Design review of the part built by this model. Coordinates are the model's own, in mm. A direction names the side the tool comes from. Round coordinates to 2 decimals unless told otherwise and drop trailing zeros. Order: outer loops, then holes, each group sorted by start corner. A loop starts at its lowest first (then second) coordinate and runs counter-clockwise, first axis right, second up. Notation, with made-up numbers: (27.5, -22.5) - (86.5, -22.5) arc R13 cw to (86.5, -3.5) - close; hole circle Ø10 at (-0.5, -25.75). An arc over 180 degrees is marked (long way). Write item = value, one per line.
from build123d import *

# Parameters (mm, degrees)
CROQUIS2_W              = 110
CROQUIS2_H              = 75
CROQUIS2_R              = 2
CROQUIS2_R_2            = 1.997516107
SALIENTE_EXTRUIR1_DEPTH = 15
CROQUIS3_R              = 4
CORTAR_EXTRUIR1_DEPTH   = 6
REDONDEO2_R             = 2
CROQUIS4_R              = 3.5
CROQUIS4_R_2            = 3
CORTAR_EXTRUIR8_DEPTH   = 15
CROQUIS5_R              = 3.701474701
SALIENTE_EXTRUIR2_DEPTH = 15
CROQUIS7_R              = 4
CROQUIS7_R_2            = 5
CORTAR_EXTRUIR9_DEPTH   = 15


with BuildPart() as part:
    # Croquis2 → Saliente-Extruir1 (new body)
    with BuildSketch(Plane.XY):
        with Locations((-693.862272549, 896.557366956)):
            Rectangle(CROQUIS2_W, CROQUIS2_H)
        with Locations((-741.862272549, 866.057366956)):
            Circle(CROQUIS2_R, mode=Mode.SUBTRACT)
        with Locations((-645.862272549, 866.057366956)):
            Circle(CROQUIS2_R, mode=Mode.SUBTRACT)
        with BuildLine():
            Line((-728.862272549, 925.057366956), (-706.362272549, 925.057366956))
            Line((-706.362272549, 925.057366956), (-681.362272549, 925.057366956))
            Line((-681.362272549, 925.057366956), (-658.862272549, 925.057366956))
            ThreePointArc((-658.862272549, 925.057366956), (-655.326738643, 923.592900862), (-653.862272549, 920.057366956))
            Line((-653.862272549, 920.057366956), (-653.862272549, 873.057366956))
            ThreePointArc((-653.862272549, 873.057366956), (-655.326738643, 869.52183305), (-658.862272549, 868.057366956))
            Line((-658.862272549, 868.057366956), (-681.362272549, 868.057366956))
            Line((-681.362272549, 868.057366956), (-706.362272549, 868.057366956))
            Line((-706.362272549, 868.057366956), (-728.862272549, 868.057366956))
            ThreePointArc((-728.862272549, 868.057366956), (-732.397806455, 869.52183305), (-733.862272549, 873.057366956))
            Line((-733.862272549, 873.057366956), (-733.862272549, 920.057366956))
            ThreePointArc((-733.862272549, 920.057366956), (-732.397806455, 923.592900862), (-728.862272549, 925.057366956))
        make_face(mode=Mode.SUBTRACT)
        with Locations((-741.862272549, 927.057366956)):
            Circle(CROQUIS2_R, mode=Mode.SUBTRACT)
        with Locations((-645.862272549, 927.057366956)):
            Circle(CROQUIS2_R_2, mode=Mode.SUBTRACT)
    extrude(amount=SALIENTE_EXTRUIR1_DEPTH)

    # Croquis3 → Cortar-Extruir1 (cut)
    with BuildSketch(Plane.XY.offset(15)):
        with Locations((-645.862272549, 927.057366956)):
            Circle(CROQUIS3_R)
        with Locations((-645.862272549, 866.057366956)):
            Circle(CROQUIS3_R)
        with Locations((-741.862272549, 866.057366956)):
            Circle(CROQUIS3_R)
        with Locations((-741.862272549, 927.057366956)):
            Circle(CROQUIS3_R)
    extrude(amount=-CORTAR_EXTRUIR1_DEPTH, mode=Mode.SUBTRACT)

    # Redondeo2
    redondeo2_edges = [part.edges().sort_by_distance(p)[0] for p in [
        (-693.862272549, 859.057366956, 15),
        (-693.862272549, 934.057366956, 15),
    ]]
    fillet(redondeo2_edges, radius=REDONDEO2_R)

    # Croquis4 → Cortar-Extruir8 (cut)
    with BuildSketch(Plane.XY.offset(15)):
        with Locations((-736.862272549, 896.557366956)):
            Circle(CROQUIS4_R)
        with Locations((-642.862272549, 896.557366956)):
            Circle(CROQUIS4_R_2)
    extrude(amount=-CORTAR_EXTRUIR8_DEPTH, mode=Mode.SUBTRACT)

    # Croquis5 → Saliente-Extruir2 (add)
    with BuildSketch(Plane.XY.offset(15)):
        with Locations((-642.862272549, 896.557366956)):
            Circle(CROQUIS5_R)
        with BuildLine():
            Line((-733.862272549, 893.78924565), (-733.862272549, 899.325488262))
            ThreePointArc((-733.862272549, 899.325488262), (-740.944244568, 896.557366956), (-733.862272549, 893.78924565))
        make_face()
    extrude(amount=-SALIENTE_EXTRUIR2_DEPTH)

    # Croquis7 → Cortar-Extruir9 (cut)
    with BuildSketch(Plane.XY.offset(15)):
        with Locations((-740.766439288, 896.084665271)):
            Circle(CROQUIS7_R)
        with Locations((-646.766439288, 896.084665271)):
            Circle(CROQUIS7_R_2)
    extrude(amount=-CORTAR_EXTRUIR9_DEPTH, mode=Mode.SUBTRACT)


solid = part.part
Item 1: Insertion check: P1, Ø4.5, axis at x = -645.86, y = 866.06, coming from the +Z side. The pin has a flat end and moves straight along its axis. Give the tip position at first contact, or say it passes through.
Data:
P1 = 9
Item 2: For faces 4 (the face through (-695, 864, 0)), 5 (the face through (-733.862, 896, 7)), 6 (the face through (-745.037, 924.623, 12.042)), list the 3-axis set-ups (+Z, -Z, +X, -X, +Y, -Y) from which the entire face can be reached by the end or side of a thin tool; tool diameter is ignored.
Data:
face_4 = -Z, +X, -X, +Y, -Y
face_5 = +Z, -Z
face_6 = +Z
Item 3: Take a section at A-A, the plane y = 905.5. State the section outline as (x, z) points, and give its area (3 significant figures).
Data:
outline = (-748.86, 0) - (-733.86, 0) - (-733.86, 15) - (-748.86, 15) - close; (-653.86, 0) - (-638.86, 0) - (-638.86, 15) - (-653.86, 15) - close
area = 450 mm2
Item 4: For line 1 along X through (y, z) = (884.5, 1); line 2 along X through (y, z) = (866.5, 9.5); line 3 along Y through (x, z) = (-675, 10.25), list the stretches that pass through material, from the lowest coordinate up. Write a range as [from, to].
Data:
line_1 = [-748.86, -733.86], [-653.86, -638.86]
line_2 = [-748.86, -745.84], [-737.89, -649.84], [-641.89, -638.86]
line_3 = [859.06, 868.06], [925.06, 934.06]
Item 5: Take a section at B-B, the plane x = -686. State the section outline as (y, z) points.
Data:
outline = (859.06, 0) - (868.06, 0) - (868.06, 15) - (861.06, 15) arc R2 ccw to (859.06, 13) - close; (925.06, 0) - (934.06, 0) - (934.06, 13) arc R2 ccw to (932.06, 15) - (925.06, 15) - close
Item 6: The part is to be moulded in two halves that separate along X. For faces 1 (the face through (-638.862, 896, 7)), 2 (the face through (-695, 859.057, 6)), 3 (the face through (-644.015, 865.291, 4.437)), say which applies: +X half, -X half, draft (parallel to the pull), parting line (faces both ways), or undercut.
Data:
face_1 = +X half
face_2 = draft
face_3 = undercut
Item 7: Take a section at C-C, the plane z = 7. State the section outline as (x, y) points, and give its area (3 significant figures).
Data:
outline = (-748.86, 859.06) - (-638.86, 859.06) - (-638.86, 934.06) - (-748.86, 934.06) - close; hole circle Ø8 at (-740.77, 896.08); hole circle Ø4 at (-741.86, 866.06); hole circle Ø4 at (-741.86, 927.06); hole (-733.86, 873.06) arc R5 ccw to (-728.86, 868.06) - (-658.86, 868.06) arc R5 ccw to (-653.86, 873.06) - (-653.86, 920.06) arc R5 ccw to (-658.86, 925.06) - (-728.86, 925.06) arc R5 ccw to (-733.86, 920.06) - close; hole circle Ø10 at (-646.77, 896.08); hole circle Ø4 at (-645.86, 866.06); hole circle Ø4 at (-645.86, 927.06)
area = 3,530 mm2
Item 8: Take a section at D-D, the plane x = -655.5. State the section outline as (y, z) points.
Data:
outline = (859.06, 0) - (869.36, 0) - (869.36, 15) - (861.06, 15) arc R2 ccw to (859.06, 13) - close; (923.76, 0) - (934.06, 0) - (934.06, 13) arc R2 ccw to (932.06, 15) - (923.76, 15) - close
